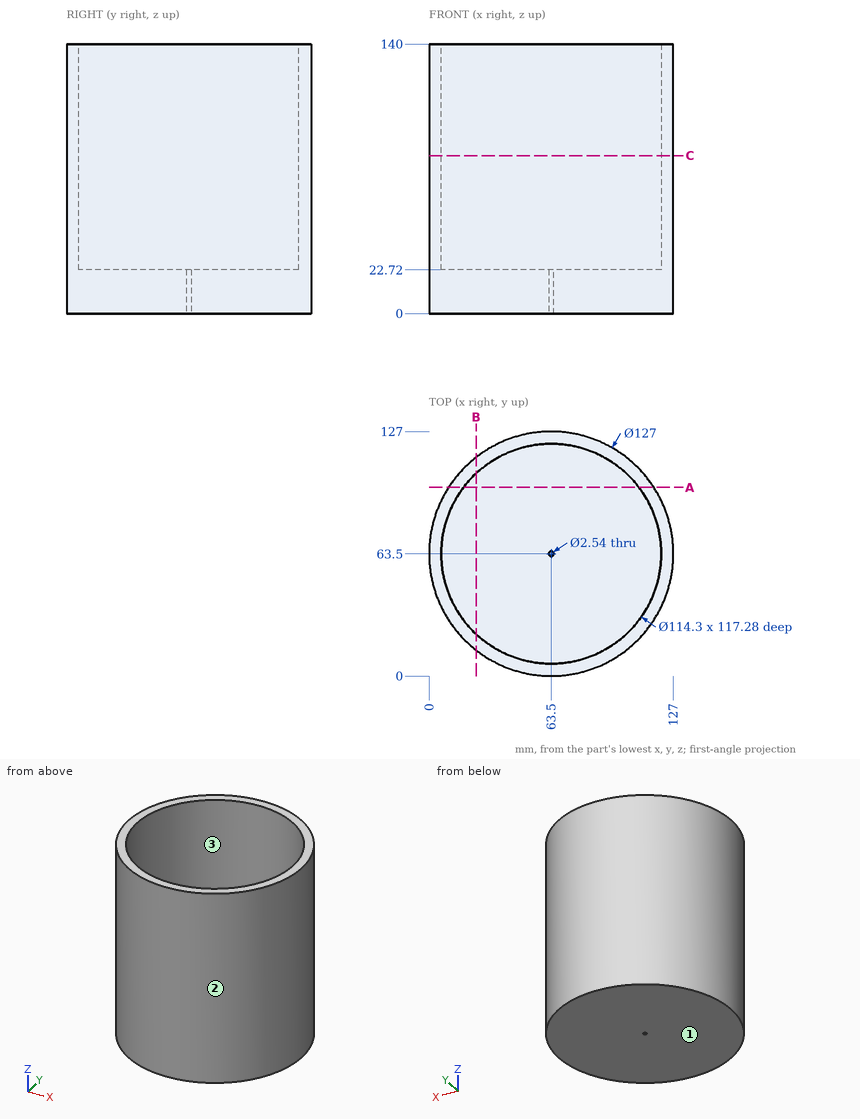
Geometry: see drawing. Coordinates: mm, zero at the bounding-box minimum. Round coordinates to 2 decimals unless told otherwise and drop trailing zeros. Loops run counter-clockwise (first coordinate to the right, second up) from the corner with the lowest first, then second, coordinate; pieces in that order, holes last. Notation, with made-up numbers: M 20.25,41.5 L 77.25,41.5 A17 ccw 77.25,49.5 Z; hole C -10.75,19.25 d6. An arc over 180 degrees is marked long. Use a Markdown table: item, result. Add a question column.
1. Ray query, line 1 along X through (y, z) = (63, 105); line 2 along Z through (x, y) = (64, 51); line 3 along X through (y, z) = (53, 70.5). Return the intervals inside material, ascending. Write a range as [from, to].
2. Pull-direction query (Y, two-part tool) for the marked faces 1, 2 and 3; classes: +Y half, -Y half, draft (parallel to the pull), parting line (faces both ways), or undercut.
3. Contact query for flat-ended pins moving along their axis: pin 1 (4 mm diameter, centred on y = 58, z = 116, fed in from +X); pin 2 (1.5 mm diameter, centred on x = 50, y = 100, fed in from +Z); pin 3 (12 mm diameter, centred on x = 102, z = 20, fed in from -Y). Output: stop coordinate, or through.
4. Cut plane B-B, the plane x = 24.5. Output: boundary loops of the cut face in (y, z).
5. Cut plane C-C, the plane z = 82. Output: boundary loops of the cut face in (x, y), and give its area (3 significant figures).
6. Cut plane A-A, the plane y = 98. Output: boundary loops of the cut face in (x, z), and give its area (3 significant figures).
Solution:
| question | item | result |
|---|---|---|
| 1 | line 1 | x = [0, 6.35], [120.65, 127] |
| 1 | line 2 | z = [0, 22.72] |
| 1 | line 3 | x = [0.87, 7.32], [119.68, 126.13] |
| 2 | face 1 | draft |
| 2 | face 2 | parting line |
| 2 | face 3 | undercut |
| 3 | pin 1 | stops at x = 126.9 |
| 3 | pin 2 | stops at z = 22.72 |
| 3 | pin 3 | stops at y = 8.95 |
| 4 | outline | M 13.39,0 L 113.61,0 L 113.61,140 L 105.27,140 L 105.27,22.72 L 21.73,22.72 L 21.73,140 L 13.39,140 Z |
| 5 | outline | C 63.5,63.5 d127; hole C 63.5,63.5 d114.3 |
| 5 | area | 2,410 mm2 |
| 6 | outline | M 10.19,0 L 116.81,0 L 116.81,140 L 109.06,140 L 109.06,22.72 L 17.94,22.72 L 17.94,140 L 10.19,140 Z |
| 6 | area | 4,240 mm2 |
